```python
from build123d import *

# Parameters (mm, degrees)
SKETCH_1_W              = 5.773502692
SKETCH_1_H              = 5
EXTRUDE_1_DEPTH         = 40
M2_2X0_45_1_D           = 1.75
M2_2X0_45_1_ON_FACE_2_D = 1.75
CUT_EXTRUDE_1_DEPTH     = 0.8
CUT_EXTRUDE_2_DEPTH     = 0.8
CHAMFER_1_SIZE          = 1


with BuildPart() as part:
    # 草图1 → 凸台-拉伸1 (new body)
    with BuildSketch(Plane(origin=(0, 0, 0), x_dir=(1, 0, 0), z_dir=(0, 1, 0))):
        Rectangle(SKETCH_1_W, SKETCH_1_H)
    extrude(amount=EXTRUDE_1_DEPTH)

    # M2.2x0.45 螺纹孔1 (through all)
    with Locations(Plane(origin=(0, 0, 0), x_dir=(0, 0, -1), z_dir=(0, -1, 0))):
        with Locations((0, 0)):
            Hole(M2_2X0_45_1_D / 2)

    # M2.2x0.45 螺纹孔1 on face 2 (through all)
    with Locations(Plane.ZX.offset(40)):
        with Locations((0, 0)):
            Hole(M2_2X0_45_1_ON_FACE_2_D / 2)

    # 草图5 → 切除-拉伸1 (cut, symmetric)
    with BuildSketch(Plane(origin=(0, 2, 0), x_dir=(-1, 0, 0), z_dir=(0, -1, 0))):
        Polygon((-2, -1.154700538), (-2, -2.5), (2, -2.5), (2, -1.154700538), (2, 1.154700538), (0, 2.309401077), (-2, 1.154700538), align=None)
    extrude(amount=CUT_EXTRUDE_1_DEPTH, both=True, mode=Mode.SUBTRACT)

    # 草图6 → 切除-拉伸2 (cut, symmetric)
    with BuildSketch(Plane(origin=(0, 38, 0), x_dir=(1, 0, 0), z_dir=(0, 1, 0))):
        Polygon((2, -2.5), (2, -1.154700538), (2, 1.154700538), (0, 2.309401077), (-2, 1.154700538), (-2, -1.154700538), (-2, -2.5), align=None)
    extrude(amount=CUT_EXTRUDE_2_DEPTH, both=True, mode=Mode.SUBTRACT)

    # 倒角1
    # the kernel refuses this chamfer: 1 mm, written as the material it takes off along each edge
    with BuildSketch(Plane(origin=(-2.886751346, -2.571682988, 2.5), x_dir=(-0.027495876610586494, 0, -0.9996219169112968), z_dir=(0, 1, 0)), Plane(origin=(2.886751346, -2.571682988, 2.5), x_dir=(-0.9996219169112965, 0, 0.027495876610591666), z_dir=(0, 1, 0))) as chamfer_1_piece_1:
        Polygon((CHAMFER_1_SIZE * 0.999621916911, -CHAMFER_1_SIZE * 0.0274958766106), (-CHAMFER_1_SIZE * 0.0274958766106, -CHAMFER_1_SIZE * 0.999621916911), (0, 0), align=None)
    extrude(amount=45.143365976, mode=Mode.SUBTRACT)
    with BuildSketch(Plane(origin=(-2.886751346, -2.571682988, -2.5), x_dir=(-0.027495876610586487, 0, 0.9996219169112968), z_dir=(0, 1, 0)), Plane(origin=(2.886751346, -2.571682988, -2.5), x_dir=(-0.9996219169112968, 0, -0.02749587661058476), z_dir=(0, 1, 0))) as chamfer_1_piece_2:
        Polygon((CHAMFER_1_SIZE * 0.999621916911, CHAMFER_1_SIZE * 0.0274958766106), (-CHAMFER_1_SIZE * 0.0274958766106, CHAMFER_1_SIZE * 0.999621916911), (0, 0), align=None)
    extrude(amount=45.143365976, mode=Mode.SUBTRACT)


solid = part.part
```
Here's how the part is built. I have some questions about the finished solid (model axes, mm). A direction names the side the tool comes from. Coordinates: 2 decimals unless noted, no trailing zeros. Order: outer loops, then holes, each group sorted by start corner. A loop starts at its lowest first (then second) coordinate and runs counter-clockwise, first axis right, second up. Notation, with made-up numbers: M -32,55.25 L -2,55.25 A18 cw -2,78.25 Z; hole C -31,-16 d11. An arc over 180 degrees is marked long. Answer as a JSON object with one key per item and string values. Group by question number.
(1) I need wall thicknesses on probe 1 along Y at (x, z) = (-1.15, 1.4); probe 2 along X at (y, z) = (13.5, 0) (3 decimals); probe 3 along Z at (x, y) = (2.5, 9). Which ranges of each line are inside material? Lowest first, please.
(2) Suppose I cut it at A-A, the plane z = 0. Please give me the cut outline in (x, y) (3 decimals).
(3) Suppose I cut it at D-D, the plane z = -1.9. Please give me the cut outline in (x, y).
(4) Which directions (+Z, -Z, +X, -X, +Y, -Y) give clear straight access to the entire face, cutting with the end or side of a thin tool? Please do faces 1 (the face through (0.99, 1.99, -1.74)), 2 (the face through (2.38, 19.72, 2.007)).
(5) If we mould it in two halves opening along Y, with no side actions, what happens to faces 3 (the face through (-1, 0, -1)), 4 (the face through (0, 38.8, 1.1)), 5 (the face through (-1, 40, -1))? For each: released by +Y, released by -Y, zero draft, split by the parting line, or undercut.
(6) For pin 1 (1.1 mm diameter, centred on x = 0, z = 0, fed in from +Y), with a flat end and sliding along its axis, tell me the tip position at first contact or that it passes through.
(7) Suppose I cut it at B-B, the plane y = 16. Please give me the cut outline in (x, z) (3 decimals).
(8) Suppose I cut it at C-C, the plane x = 0.5. Please give me the cut outline in (y, z).
Values found:
{
 "1": {"probe 1": "y = 0 to 1.2, 2.8 to 37.2, 38.8 to 40", "probe 2": "x = -2.887 to -0.875, 0.875 to 2.887", "probe 3": "z = -1.89 to 1.89"},
 "2": {"outline": "M -2.887,0 L -0.875,0 L -0.875,1.2 L -2,1.2 L -2,2.8 L -0.875,2.8 L -0.875,37.2 L -2,37.2 L -2,38.8 L -0.875,38.8 L -0.875,40 L -2.887,40 Z; M 0.875,0 L 2.887,0 L 2.887,40 L 0.875,40 L 0.875,38.8 L 2,38.8 L 2,37.2 L 0.875,37.2 L 0.875,2.8 L 2,2.8 L 2,1.2 L 0.875,1.2 Z"},
 "3": {"outline": "M -2.49,0 L 2.49,0 L 2.49,40 L -2.49,40 Z; hole M -0.71,1.2 L 0.71,1.2 L 0.71,2.8 L -0.71,2.8 Z; hole M -0.71,37.2 L 0.71,37.2 L 0.71,38.8 L -0.71,38.8 Z"},
 "4": {"face 1": "+Z", "face 2": "+Z, +X, +Y, -Y"},
 "5": {"face 3": "released by -Y", "face 4": "undercut", "face 5": "released by +Y"},
 "6": {"pin 1": "passes through"},
 "7": {"outline": "M -2.887,-1.5 L -1.887,-2.5 L 1.887,-2.5 L 2.887,-1.5 L 2.887,1.5 L 1.887,2.5 L -1.887,2.5 L -2.887,1.5 Z; hole C 0,0 d1.75"},
 "8": {"outline": "M 0,-2.5 L 40,-2.5 L 40,-0.72 L 38.8,-0.72 L 38.8,-2.02 L 37.2,-2.02 L 37.2,-0.72 L 2.8,-0.72 L 2.8,-2.02 L 1.2,-2.02 L 1.2,-0.72 L 0,-0.72 Z; M 0,0.72 L 1.2,0.72 L 1.2,2.5 L 0,2.5 Z; M 2.8,0.72 L 37.2,0.72 L 37.2,2.5 L 2.8,2.5 Z; M 38.8,0.72 L 40,0.72 L 40,2.5 L 38.8,2.5 Z"}
}
